Could you check a few things on this model? Use its own coordinates, in mm. A direction names the side the tool comes from. Give positions to 0.01 mm unless a question says otherwise; leave off trailing zeros. Order: outer loops, then holes, each group sorted by start corner. A loop starts at its lowest first (then second) coordinate and runs counter-clockwise, first axis right, second up.
from build123d import *

# Parameters (mm, degrees)
ESQUISSE1_R        = 2
BOSS_EXTRU_1_DEPTH = 5
BOSS_EXTRU_2_DEPTH = 7.5
BOSS_EXTRU_3_DEPTH = 2.5
BOSS_EXTRU_4_START = 5
ESQUISSE5_R        = 2
BOSS_EXTRU_4_DEPTH = 5
ESQUISSE6_W        = 5
ESQUISSE6_H        = 5
BOSS_EXTRU_5_DEPTH = 2.5


with BuildPart() as part:
    # Esquisse1 → Boss.-Extru.1 (new body)
    with BuildSketch(Plane(origin=(0, 0, 0), x_dir=(1, 0, 0), z_dir=(0, 1, 0))):
        with Locations(Location((0, 0, 0), (0, 0, 270))):
            Circle(ESQUISSE1_R)
    extrude(amount=BOSS_EXTRU_1_DEPTH)

    # Esquisse2 → Boss.-Extru.2 (add)
    with BuildSketch(Plane(origin=(0, 5, 0), x_dir=(1, 0, 0), z_dir=(0, 1, 0))):
        with BuildLine():
            ThreePointArc((2, 0), (-0.157353741, 1.993800341), (-1.9752398, -0.313731942))
            add(Edge.make_bspline(
                [(-1.9752398, -0.313731942), (6.018007313, -27.755724693), (31.670728762, -44.785499484)],
                knots=[0, 0, 0, 1, 1, 1], degree=2))
            add(Edge.make_bspline(
                [(2, 0), (7.431064096, -26.884767596), (31.670728762, -44.785499484)],
                knots=[0, 0, 0, 1, 1, 1], degree=2))
        make_face()
    extrude(amount=BOSS_EXTRU_2_DEPTH)

    # Esquisse4 → Boss.-Extru.3 (add)
    with BuildSketch(Plane.XZ):
        Polygon((-0.480726256, 9.001048314), (0.480719689, 9.001048314), (1.384199773, 4.71416076), (4.461921977, 7.832061849), (5.270741775, 7.312264927), (3.713131196, 3.217447416), (7.987940467, 4.176450473), (8.387339547, 3.301888479), (4.863168658, 0.699216639), (8.977843256, -0.805155029), (8.841015231, -1.756814841), (4.46918339, -2.041011092), (7.117343203, -5.53113011), (6.487730005, -6.257742475), (2.65626293, -4.133232834), (2.99713593, -8.501011074), (2.0746353, -8.771881699), (-3.284e-06, -4.913182966), (-2.074641867, -8.771881699), (-2.997142497, -8.501011074), (-2.656269497, -4.133232834), (-6.487736572, -6.257742475), (-7.11734977, -5.53113011), (-4.469189957, -2.041011092), (-8.841021798, -1.756814841), (-8.977849823, -0.805155029), (-4.863175225, 0.699216639), (-8.387346114, 3.301888479), (-7.987947034, 4.176450473), (-3.713137763, 3.217447416), (-5.270748343, 7.312264927), (-4.461928544, 7.832061849), (-1.38420634, 4.71416076), align=None)
    extrude(amount=BOSS_EXTRU_3_DEPTH)

    # Esquisse5 → Boss.-Extru.4 (add)
    with BuildSketch(Plane.XZ.offset(2.5).offset(BOSS_EXTRU_4_START)):
        with Locations(Location((0, 0, 0), (0, 0, 270))):
            Circle(ESQUISSE5_R)
    extrude(amount=-BOSS_EXTRU_4_DEPTH)

    # Esquisse6 → Boss.-Extru.5 (add)
    with BuildSketch(Plane.XZ.offset(7.5)):
        Rectangle(ESQUISSE6_W, ESQUISSE6_H)
    extrude(amount=BOSS_EXTRU_5_DEPTH)


solid = part.part
Item 1: Imagine slicing it at B-B on y = 1.5. List the corners of the cut face in (x, z) for me.
Findings:
outline: circle Ø4 at (0, 0)
Item 2: For faces 4 (the flat face through (6.65, -1.23, 2.02)), 5 (the flat face through (0, -9, -2.5)), 6 (the flat face through (-2, -2.5, -2)), 7 (the flat face through (2.824, -1.232, -6.287)), which set-ups out of +Z, -Z, +X, -X, +Y, -Y let a thin tool reach every point of the face, with its end or its side?
Findings:
face 4: +X, +Y, -Y
face 5: -Z, +X, -X, -Y
face 6: none
face 7: +Y, -Y
Item 3: Please list where these lines run through material, in increasing order: line 1 along Y through (x, z) = (1, 6); line 2 along Y through (x, z) = (2.5, 7.5); line 3 along X through (y, z) = (3.75, 0).
Findings:
line 1: y = -2.5 to 0, 5 to 12.5
line 2: y = 5 to 12.5
line 3: x = -2 to 2
Item 4: We'd pull the mould along Z, two halves only. Please class faces 1 (the flat face through (-5.81, -1.23, -3.81)), 2 (the flat face through (0.926, -1.232, 6.888)), 3 (the flat face through (2.5, -9, 0)): +Z half, -Z half, draft (parallel to the pull), parting line (faces both ways), or undercut.
Findings:
face 1: undercut
face 2: +Z half
face 3: draft
Item 5: For pin 1 (12 mm diameter, centred on y = 6, z = 6, fed in from +X); pin 2 (2 mm diameter, centred on x = 1, y = -9, fed in from +Z); pin 3 (0.8 mm diameter, centred on x = 0, y = -1, fed in from +Z); pin 4 (5.5 mm diameter, centred on x = 3.5, z = -2.5, fed in from -Y), each with a flat end and sliding along its axis, tell me the tip position at first contact or that it passes through.
Findings:
pin 1: stops at x = 5.54
pin 2: stops at z = 2.5
pin 3: stops at z = 9
pin 4: stops at y = -10
